Here's how the part is built. I have some questions about the finished solid (model axes, mm). Face numbers are marked on the shaded views. A direction names the side the tool comes from. Coordinates: 2 decimals unless noted, no trailing zeros. Write each loop counter-clockwise with the first axis right and the second up, starting at its lowest first coordinate (ties: lowest second). Pieces come first, ordered by that corner, then holes. Notation, with made-up numbers: (78, 33) -> (99, 33) arc R17 cw to (99, 38) -> close; hole circle Ø8 at (11, 85.5). An arc over 180 degrees is marked (long way). Put each result on its own line as item: value. Start each with the question number.
Item 1: If we mould it in two halves opening along Z, with no side actions, what happens to the marked faces 1, 2, 3 and 4? For each: released by +Z, released by -Z, zero draft, split by the parting line, or undercut.
Item 2: I need wall thicknesses on line 1 (Z direction, x = -64, y = 4.5); line 2 (Y direction, x = -73.05, z = -45); line 3 (X direction, y = 4.5, z = -0.5). Which ranges of each line are inside material? Lowest first, please. Write a range as [from, to].
Item 3: I want a section at A-A, the plane z = 8. List the corners of the cut face in (x, y) for me, then the cut area to 3 significant figures.
Item 4: For pin 1 (10 mm diameter, centred on x = -65, y = 0.5, fed in from -Z); pin 2 (3.5 mm diameter, centred on y = -2, z = -17, fed in from -X); pin 3 (1.5 mm diameter, centred on y = -2.5, z = 5.5, fed in from -X); pin 4 (6 mm diameter, centred on x = -63, y = -4, fed in from +Z), each with a flat end and sliding along its axis, tell me the tip position at first contact or that it passes through.
Item 5: On a 3-axis mill with a long thin cutter (end or side, diameter ignored), from which of +Z, -Z, +X, -X, +Y, -Y can I reach the whole of each face in a straight line? I mean the marked faces 5, 6 and 7. Say none if no direction works.
Item 6: I want a section at C-C, the plane z = -18.5. List the corners of the cut face in (x, y) for me, then the cut area to 3 significant figures.
Item 7: I want a section at B-B, the plane x = -65.5. List the corners of the cut face in (y, z) for me.
Item 8: I want a section at D-D, the plane y = -7.5. List the corners of the cut face in (x, z) for me.
from build123d import *

# Parameters (mm, degrees)
SKETCH_1_W          = 30
SKETCH_1_H          = 20
EXTRUDE_1_DEPTH     = 3
EXTRUDE_2_DEPTH     = 40
SKETCH_1_4_W        = 3.5
SKETCH_1_4_H        = 20
EXTRUDE_3_DEPTH     = 40
SKETCH_3_R          = 6
CUT_EXTRUDE_2_DEPTH = 38
SKETCH_4_R          = 6
SKETCH_4_R_2        = 5.5
EXTRUDE_4_DEPTH     = 1
SKETCH_5_R          = 6
SKETCH_5_R_2        = 5.5
EXTRUDE_5_DEPTH     = 1
SKETCH_7_W          = 3.5
SKETCH_7_H          = 20
EXTRUDE_6_DEPTH     = 23
SKETCH_9_W          = 20
SKETCH_9_H          = 20
SKETCH_9_R          = 1.5
EXTRUDE_7_DEPTH     = 3


with BuildPart() as part:
    # Sketch 1 → Extrude 1 (new body)
    with BuildSketch(Plane.XY):
        with Locations((-68, -0.145751311)):
            Rectangle(SKETCH_1_W, SKETCH_1_H)
    extrude(amount=EXTRUDE_1_DEPTH)

    # Sketch 1_3 → Extrude 2 (add)
    with BuildSketch(Plane.XY):
        Polygon((-56.5, 9.854248689), (-56.5, -10.145751311), (-53, -10.145751311), (-53, -0.145751311), (-53, 9.854248689), align=None)
    extrude(amount=-EXTRUDE_2_DEPTH)

    # Sketch 1_4 → Extrude 3 (add)
    with BuildSketch(Plane.XY):
        with Locations((-81.25, -0.145751311)):
            Rectangle(SKETCH_1_4_W, SKETCH_1_4_H)
    extrude(amount=-EXTRUDE_3_DEPTH)

    # Sketch 3 → Cut-Extrude 2 (cut)
    with BuildSketch(Plane.ZY.offset(83)):
        with Locations((-18.5, -0.145751311)):
            Circle(SKETCH_3_R)
    extrude(amount=-CUT_EXTRUDE_2_DEPTH, mode=Mode.SUBTRACT)

    # Sketch 4 → Extrude 4 (add)
    with BuildSketch(Plane(origin=(-56.5, 0, 0), x_dir=(0, 0, -1), z_dir=(1, 0, 0))):
        with Locations((18.5, -0.145751311)):
            Circle(SKETCH_4_R)
        with Locations((18.5, -0.145751311)):
            Circle(SKETCH_4_R_2, mode=Mode.SUBTRACT)
    extrude(amount=EXTRUDE_4_DEPTH)

    # Sketch 5 → Extrude 5 (add)
    with BuildSketch(Plane(origin=(-79.5, 0, 0), x_dir=(0, 0, -1), z_dir=(1, 0, 0))):
        with Locations((18.5, -0.145751311)):
            Circle(SKETCH_5_R)
        with Locations((18.5, -0.145751311)):
            Circle(SKETCH_5_R_2, mode=Mode.SUBTRACT)
    extrude(amount=-EXTRUDE_5_DEPTH)

    # Sketch 7 → Extrude 6 (add)
    with BuildSketch(Plane(origin=(-79.5, 0, 0), x_dir=(0, 0, -1), z_dir=(1, 0, 0))):
        with Locations((38.25, -0.145751311)):
            Rectangle(SKETCH_7_W, SKETCH_7_H)
    extrude(amount=EXTRUDE_6_DEPTH)

    # Sketch 9 → Extrude 7 (add)
    with BuildSketch(Plane.ZY.offset(71)):
        with Locations((-50, -0.145751311)):
            Rectangle(SKETCH_9_W, SKETCH_9_H)
        with Locations((-55, 0.144248689)):
            Circle(SKETCH_9_R, mode=Mode.SUBTRACT)
        with Locations((-45, 0.144248689)):
            Circle(SKETCH_9_R, mode=Mode.SUBTRACT)
    extrude_7 = extrude(amount=EXTRUDE_7_DEPTH)

    # Mirror 1: Extrude 7 across plane
    add(extrude_7.mirror(Plane.XY.offset(-18.5)))


solid = part.part
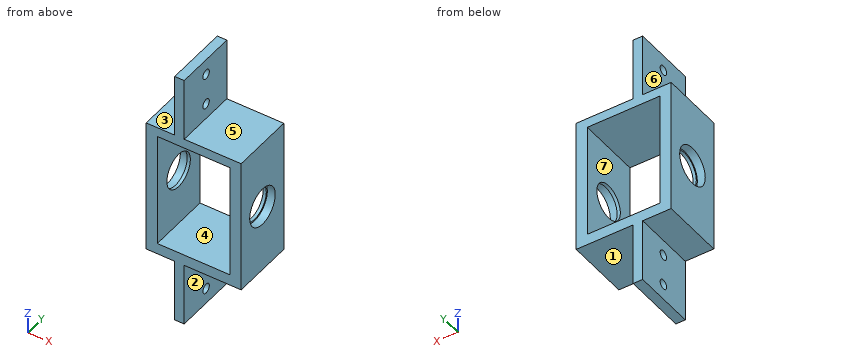
Calculated:
1. face 1: released by -Z
1. face 2: zero draft
1. face 3: released by +Z
1. face 4: undercut
2. line 1: z = [-40, -36.5], [0, 3]
2. line 2: y = [-10.15, -1.36], [1.64, 9.85]
2. line 3: x = [-83, -79.5], [-56.5, -53]
3. outline: (-74, -10.15) -> (-71, -10.15) -> (-71, -1.36) -> (-74, -1.36) -> close; (-74, 1.64) -> (-71, 1.64) -> (-71, 9.85) -> (-74, 9.85) -> close
3. area: 51.0 mm2
4. pin 1: stops at z = -40
4. pin 2: passes through
4. pin 3: stops at x = -74
4. pin 4: stops at z = 3
5. face 5: +Z, +X, +Y, -Y
5. face 6: +Z, -X, +Y, -Y
5. face 7: +Y, -Y
6. outline: (-83, -10.15) -> (-79.5, -10.15) -> (-79.5, -5.65) -> (-80.5, -5.65) -> (-80.5, -6.15) -> (-83, -6.15) -> close; (-83, 5.85) -> (-80.5, 5.85) -> (-80.5, 5.35) -> (-79.5, 5.35) -> (-79.5, 9.85) -> (-83, 9.85) -> close; (-56.5, -10.15) -> (-53, -10.15) -> (-53, -6.15) -> (-55.5, -6.15) -> (-55.5, -5.65) -> (-56.5, -5.65) -> close; (-56.5, 5.35) -> (-55.5, 5.35) -> (-55.5, 5.85) -> (-53, 5.85) -> (-53, 9.85) -> (-56.5, 9.85) -> close
6. area: 58.0 mm2
7. outline: (-10.15, -40) -> (9.85, -40) -> (9.85, -36.5) -> (-10.15, -36.5) -> close; (-10.15, 0) -> (9.85, 0) -> (9.85, 3) -> (-10.15, 3) -> close
8. outline: (-83, -40) -> (-74, -40) -> (-74, -60) -> (-71, -60) -> (-71, -40) -> (-53, -40) -> (-53, 3) -> (-71, 3) -> (-71, 23) -> (-74, 23) -> (-74, 3) -> (-83, 3) -> close; hole (-79.5, -36.5) -> (-56.5, -36.5) -> (-56.5, 0) -> (-79.5, 0) -> close
